Autodesk Inventor part; units mm, degrees
ref_plane "YZ Plane" through (0, 0, 0) normal (1, 0, 0) x (0, 1, 0)
ref_plane "XZ Plane" through (0, 0, 0) normal (0, 1, 0) x (-1, 0, 0)
ref_plane "XY Plane" through (0, 0, 0) normal (0, 0, 1) x (1, 0, 0)
sketch "Sketch1" plane through (0, 0, 0) normal (0, 1, 0) x (-1, 0, 0)
  line L0 (-9.9, 4.7) -> (9.9, 4.7)
  line L1 (9.9, 4.7) -> (9.9, -4.7)
  line L2 (9.9, -4.7) -> (-9.9, -4.7)
  line L3 (-9.9, -4.7) -> (-9.9, 4.7)
  line L4 (-9.9, 4.7) -> (9.9, -4.7) construction
  line L5 (9.9, 4.7) -> (-9.9, -4.7) construction
  line L6 (12.5, -5.4) -> (-6.5, -5.4)
  line L7 (-6.5, -5.4) -> (-6.5, -4.9)
  line L8 (-6.5, -4.9) -> (12.5, -4.9)
  line L9 (12.5, -4.9) -> (12.5, -5.4)
  line L10 (-6.5, -5.4) -> (-7, -5.4)
  line L11 (-7, -5.4) -> (-7, -4.7)
  line L12 (-7, -4.7) -> (-6.5, -4.7)
  line L13 (-6.5, -4.7) -> (-6.5, -5.4)
  arc A0 (12.5, -5.4) -> (9.8, -5.4) centre (11.15, -5.4) ccw construction
  arc A1 (9.8, -5.4) -> (12.5, -5.4) centre (11.15, -5.4) ccw
  point P0 (0, 0)
  point P1 (-7, -5.05)
  dimension "d0" = 19.8
  dimension "d1" = 9.4
  dimension "d2" = 0.5
  dimension "d3" = 0.5
  dimension "d4" = 0.7
  dimension "d5" = 19
  dimension "d6" = 2.7
  dimension "d7" = 2.9
extrude "Extrusion1" add sketch "Sketch1" along normal blind 6.4
sketch "Sketch3" plane through (-9.9, 0, 4.7) normal (0, 0, 1) x (1, 0, 0)
  line L0 (0, 3) -> (3.1, 3)
  line L1 (3.1, 3) -> (3.1, 3.4)
  line L2 (3.1, 3.4) -> (0, 3.4)
  line L3 (0, 3.4) -> (0, 3)
  line L4 (7.7, 3) -> (10.8, 3)
  line L5 (10.8, 3) -> (10.8, 3.4)
  line L6 (10.8, 3.4) -> (7.7, 3.4)
  line L7 (7.7, 3.4) -> (7.7, 3)
  line L8 (16.7, 3.4) -> (19.8, 3.4)
  line L9 (19.8, 3.4) -> (19.8, 3)
  line L10 (19.8, 3) -> (16.7, 3)
  line L11 (16.7, 3) -> (16.7, 3.4)
  line L12 (-2.6, 6.4) -> (16.4, 6.4)
  line L13 (19.8, 0) -> (16.9, 0)
  line L14 (-2.6, 6.4) -> (19.8, 0) construction
  line L15 (19.8, 0) -> (19.8, 6.4)
  line L16 (0, 0) -> (0, 6.4)
  point P0 (9.9, 0)
  point P1 (0, 3.2)
  point P2 (8.6, 3.2)
  point P3 (19.8, 3.2)
  dimension "d10" = 3.1
  dimension "d11" = 0.4
  dimension "d12" = 9
extrude "Extrusion2" add sketch "Sketch3" along normal blind 4.9
sketch "Sketch4" plane through (0, 6.4, 0) normal (0, 1, 0) x (1, 0, 0)
  line L0 (-12.5, 5.4) -> (-12.5, 4.9)
  line L1 (-12.5, 4.9) -> (6.5, 4.9)
  line L2 (6.5, 4.9) -> (6.5, 4.7)
  line L3 (6.5, 4.7) -> (-9.9, 4.7)
  line L4 (-9.9, 4.7) -> (-9.9, -4.7)
  line L5 (-9.9, -4.7) -> (9.9, -4.7)
  line L6 (9.9, -4.7) -> (9.9, 4.7)
  line L7 (9.9, 4.7) -> (7, 4.7)
  line L8 (7, 4.7) -> (7, 5.4)
  line L9 (7, 5.4) -> (-9.8, 5.4)
  arc A0 (-9.8, 5.4) -> (-12.5, 5.4) centre (-11.15, 5.4) ccw
  line L10 (6.5, 4.9) -> (6.5, 4.7)
  line L11 (6.5, 4.7) -> (7, 4.7)
  point P0 (0, 0)
extrude "Extrusion3" cut sketch "Sketch4" against normal blind 0.1 contours A0 L9 L8 L11 L2 L1 L0
sketch "Sketch5" plane through (0, 0, 0) normal (0, -1, 0) x (1, 0, 0)
  line L0 (-12.5, -5.4) -> (-12.5, -4.9)
  arc A0 (-12.5, -5.4) -> (-9.8, -5.4) centre (-11.15, -5.4) ccw
  line L1 (7, -5.4) -> (-9.8, -5.4)
  line L2 (7, -4.7) -> (7, -5.4)
  line L3 (9.9, -4.7) -> (7, -4.7)
  line L4 (9.9, 4.7) -> (9.9, -4.7)
  line L5 (-9.9, 4.7) -> (9.9, 4.7)
  line L6 (-9.9, -4.7) -> (-9.9, 4.7)
  line L7 (6.5, -4.7) -> (-9.9, -4.7)
  line L8 (6.5, -4.9) -> (6.5, -4.7)
  line L9 (-12.5, -4.9) -> (6.5, -4.9)
  line L10 (7, -4.7) -> (6.5, -4.7)
  line L11 (7, -4.7) -> (6.5, -4.7)
  point P0 (0, 0)
extrude "Extrusion4" cut sketch "Sketch5" against normal blind 0.1 contours L0 L9 L8 L10 L2 L1 A0
sketch "Sketch6" plane through (0, 6.4, 0) normal (0, 1, 0) x (1, 0, 0)
  circle A0 centre (-4.75, -1.8) radius 1.175
  circle A1 centre (4.75, -1.8) radius 1.175
  line L0 (-4.75, -1.8) -> (4.75, -1.8) construction
  line L1 (-9.9, -4.7) -> (9.9, -4.7)
  point P0 (0, 0)
  point P1 (0, -1.8)
  dimension "d19" = 2.35
  dimension "d20" = 9.5
  dimension "d21" = 2.9
extrude "Extrusion5" cut sketch "Sketch6" against normal up to surface (6.4 mm away)
sketch "Sketch7" plane through (0, 6.3, 0) normal (0, 1, 0) x (1, 0, 0)
  line L0 (6.5, 4.7) -> (6.5, 4.9)
  line L1 (7, 4.7) -> (6.5, 4.7)
  line L2 (7, 5.4) -> (7, 4.7)
  line L3 (-9.8, 5.4) -> (7, 5.4)
  arc A0 (-9.8, 5.4) -> (-12.5, 5.4) centre (-11.15, 5.4) ccw
  line L4 (-12.5, 4.9) -> (-12.5, 5.4)
  line L5 (6.5, 4.9) -> (-12.5, 4.9)
  point P0 (0, 0)
extrude "Extrusion6" cut sketch "Sketch7" against normal blind 1
sketch "Sketch8" plane through (0, 0.1, 0) normal (0, -1, 0) x (1, 0, 0)
  line L0 (6.5, -4.7) -> (7, -4.7)
  line L1 (6.5, -4.9) -> (6.5, -4.7)
  line L2 (-12.5, -4.9) -> (6.5, -4.9)
  line L3 (-12.5, -5.4) -> (-12.5, -4.9)
  arc A0 (-12.5, -5.4) -> (-9.8, -5.4) centre (-11.15, -5.4) ccw
  line L4 (7, -5.4) -> (-9.8, -5.4)
  line L5 (7, -4.7) -> (7, -5.4)
  point P0 (0, 0)
extrude "Extrusion7" cut sketch "Sketch8" against normal blind 1
properties part number "LimitSwitch_V1" material "Acetal Resin, Black"
Could you check a few things on this model? Use its own coordinates, in mm. A direction names the side the tool comes from. Coordinates: 2 decimals unless noted, no trailing zeros. Order: outer loops, then holes, each group sorted by start corner. A loop starts at its lowest first (then second) coordinate and runs counter-clockwise, first axis right, second up. Notation, with made-up numbers: (-1.75, 86.5) -> (54.25, 86.5) arc R27 ccw to (54.25, 112.5) -> close; hole circle Ø11 at (34.5, -21). An arc over 180 degrees is marked (long way). One line per question, with ' | ' between items.
Q1. I'm going to push flat-ended pins straight in: P1, Ø1.6, axis at x = 0, z = 7, coming from the +Y side; P2, Ø1.5, axis at x = -5, y = 2, coming from the +Z side; P3, Ø0.9, axis at x = -0.5, z = 6.5, coming from the -Y side. Where does each tip first touch, or does it pass through?
Return value:
P1: y = 3.4 | P2: z = 4.7 | P3: y = 3
Q2. Thinking about a two-plate mould opening in Z: for faces 1 (the face through (-8, 3, 7)), 2 (the face through (-5.682, 3.245, 2.515)), 3 (the face through (-11.18, 3.17, -6.75)), which applies, pulls with the +Z half, pulls with the -Z half, needs draft (parallel to the pull), parting line crosses it, or undercut?
Return value:
face 1: needs draft | face 2: undercut | face 3: pulls with the -Z half
Q3. Imagine slicing it at B-B on y = 2.5. Please give me the cut outline in (x, z) (3 decimals).
Return value:
outline: (-12.5, -5.4) arc R1.35 ccw to (-9.8, -5.4) -> (7, -5.4) -> (7, -4.7) -> (9.9, -4.7) -> (9.9, 4.7) -> (-9.9, 4.7) -> (-9.9, -4.7) -> (6.5, -4.7) -> (6.5, -4.9) -> (-12.5, -4.9) -> close; hole circle Ø2.35 at (-4.75, 1.8); hole circle Ø2.35 at (4.75, 1.8)
Q4. Imagine slicing it at A-A on x = -6.25. Please give me the cut outline in (y, z), and give its area (3 significant figures).
Return value:
outline: (0, -4.7) -> (6.4, -4.7) -> (6.4, 4.7) -> (0, 4.7) -> close; (1.1, -5.4) -> (5.3, -5.4) -> (5.3, -4.9) -> (1.1, -4.9) -> close | area: 62.3 mm²
Q5. On a 3-axis mill with a long thin cutter (end or side, diameter ignored), from which of +Z, -Z, +X, -X, +Y, -Y can I reach the whole of each face in a straight line? I mean faces 4 (the face through (-3, 3, -4.9)), 5 (the face through (-8, 3.4, 7)), 6 (the face through (-9.9, 3, 1)), 7 (the face through (8, 3, 7)), 8 (the face through (-2, 3, -5.4)). Say none if no direction works.
Return value:
face 4: -X, +Y, -Y | face 5: +Z, +X, -X, +Y | face 6: +Z, -X, +Y, -Y | face 7: +Z, +X, -X, -Y | face 8: -Z, +X, +Y, -Y
Q6. If I drill on L1, parallel to Z at x = 4.75, y = 2.75 (3 decimals); L2, parallel to X at y = 3.75, z = 1.8 (3 decimals); L3, parallel to Z at x = -1, y = 1.5, over which ranges is the centre line in solid material (lowest first)?
Return value:
L1: -5.4 to -4.9, -4.7 to 0.625, 2.975 to 4.7 | L2: -9.9 to -5.925, -3.575 to 3.575, 5.925 to 9.9 | L3: -5.4 to -4.9, -4.7 to 4.7
Q7. Imagine slicing it at D-D on x = 4.75. Please give me the cut outline in (y, z) (3 decimals).
Return value:
outline: (0, -4.7) -> (6.4, -4.7) -> (6.4, 0.625) -> (0, 0.625) -> close; (0, 2.975) -> (6.4, 2.975) -> (6.4, 4.7) -> (0, 4.7) -> close; (1.1, -5.4) -> (5.3, -5.4) -> (5.3, -4.9) -> (1.1, -4.9) -> close
Q8. Imagine slicing it at C-C on z = 1.8. Please give me the cut outline in (x, y) (3 decimals).
Return value:
outline: (-9.9, 0) -> (-5.925, 0) -> (-5.925, 6.4) -> (-9.9, 6.4) -> close; (-3.575, 0) -> (3.575, 0) -> (3.575, 6.4) -> (-3.575, 6.4) -> close; (5.925, 0) -> (9.9, 0) -> (9.9, 6.4) -> (5.925, 6.4) -> close
